from build123d import *

# Parameters (mm, degrees)
EXTRUDE1_DEPTH = 78
FILLET1_R      = 20
FILLET2_R      = 10
SKETCH3_R      = 7.5
EXTRUDE3_DEPTH = 6
FILLET3_R      = 30
SKETCH4_W      = 276.639181173
SKETCH4_H      = 310.570393871
EXTRUDE4_DEPTH = 79
SKETCH5_W      = 173
SKETCH5_H      = 59
EXTRUDE5_DEPTH = 65
EXTRUDE6_DEPTH = 94
SKETCH2_R      = 5
EXTRUDE2_DEPTH = 405
FILLET4_R      = 30
FILLET5_R      = 30


with BuildPart() as part:
    # Sketch1 → Extrude1 (new body)
    with BuildSketch(Plane(origin=(0, 0, 0), x_dir=(0, 0, -1), z_dir=(1, 0, 0))):
        Polygon((-38.878108718, 93.787762145), (-38.878108718, 8.787762145), (16.121891282, -76.212237855), (361.121891282, -76.212237855), (361.121891282, 123.787762145), (356.121891282, 123.787762145), (356.121891282, -71.212237855), (17.886597165, -71.212237855), (-33.878108718, 8.787762145), (-33.878108718, 93.787762145), align=None)
    extrude(amount=EXTRUDE1_DEPTH)

    # Fillet1
    fillet1_edges = [part.edges().sort_by_distance(p)[0] for p in [
        (39, -71.212237855, -356.121891282),
        (39, -76.212237855, -361.121891282),
    ]]
    fillet(fillet1_edges, radius=FILLET1_R)

    # Fillet2
    fillet2_edges = [part.edges().sort_by_distance(p)[0] for p in [
        (39, 8.787762145, 33.878108718),
        (39, -71.212237855, -17.886597165),
        (39, -76.212237855, -16.121891282),
        (39, 8.787762145, 38.878108718),
    ]]
    fillet(fillet2_edges, radius=FILLET2_R)

    # Sketch3 → Extrude3 (cut, through all)
    with BuildSketch(Plane(origin=(0, -71.212237855, 0), x_dir=(1, 0, 0), z_dir=(0, 1, 0))):
        with Locations((37.276272586, 74.00186583)):
            Circle(SKETCH3_R)
    extrude(amount=-EXTRUDE3_DEPTH, mode=Mode.SUBTRACT)

    # Fillet3
    fillet3_edges = [part.edges().sort_by_distance(p)[0] for p in [
        (0, 93.787762145, 36.378108718),
        (78, 93.787762145, 36.378108718),
    ]]
    fillet(fillet3_edges, radius=FILLET3_R)

    # Sketch4 → Extrude4 (cut, through all)
    with BuildSketch(Plane(origin=(78, 0, 0), x_dir=(0, 0, -1), z_dir=(1, 0, 0))):
        with Locations((344.441481869, 21.193022351)):
            Rectangle(SKETCH4_W, SKETCH4_H)
    extrude(amount=-EXTRUDE4_DEPTH, mode=Mode.SUBTRACT)

    # Sketch5 → Extrude5 (add)
    with BuildSketch(Plane(origin=(0, 0, -206.121891282), x_dir=(-1, 0, 0), z_dir=(0, 0, -1))):
        with Locations((-39, -46.712237855)):
            Rectangle(SKETCH5_W, SKETCH5_H)
    extrude(amount=EXTRUDE5_DEPTH)

    # Sketch6 → Extrude6 (add)
    with BuildSketch(Plane(origin=(0, 0, -271.121891282), x_dir=(-1, 0, 0), z_dir=(0, 0, -1))):
        with BuildLine():
            Line((-125.5, -76.212237855), (47.5, -76.212237855))
            Line((47.5, -76.212237855), (47.5, 101.787762145))
            ThreePointArc((47.5, 101.787762145), (32.855339059, 137.143101205), (-2.5, 151.787762145))
            Line((-2.5, 151.787762145), (-75.5, 151.787762145))
            ThreePointArc((-75.5, 151.787762145), (-110.855339059, 137.143101205), (-125.5, 101.787762145))
            Line((-125.5, 101.787762145), (-125.5, -76.212237855))
        make_face()
    extrude(amount=EXTRUDE6_DEPTH)

    # Sketch2 → Extrude2 (cut, through all)
    with BuildSketch(Plane.XY.offset(38.878108718)):
        with Locations((39, 78.787762145)):
            Circle(SKETCH2_R)
    extrude(amount=-EXTRUDE2_DEPTH, mode=Mode.SUBTRACT)

    # Fillet4
    fillet4_edges = [part.edges().sort_by_distance(p)[0] for p in [
        (125.5, -17.212237855, -238.621891282),
        (39, -17.212237855, -206.121891282),
        (-47.5, -17.212237855, -238.621891282),
        (39, -17.212237855, -271.121891282),
        (125.5, 42.287762145, -271.121891282),
        (-47.5, 42.287762145, -271.121891282),
        (-32.855339059, 137.143101205, -271.121891282),
        (39, 151.787762145, -271.121891282),
        (110.855339059, 137.143101205, -271.121891282),
    ]]
    fillet(fillet4_edges, radius=FILLET4_R)

    # Fillet5
    fillet5_edges = [part.edges().sort_by_distance(p)[0] for p in [
        (125.5, 12.787762145, -365.121891282),
        (39, -76.212237855, -365.121891282),
        (-47.5, 12.787762145, -365.121891282),
        (-32.855339059, 137.143101205, -365.121891282),
        (39, 151.787762145, -365.121891282),
        (110.855339059, 137.143101205, -365.121891282),
    ]]
    fillet(fillet5_edges, radius=FILLET5_R)


solid = part.part
Can you work these out from the model? Positions are in its coordinate system, mm. A direction names the side the tool comes from. Give positions to 0.01 mm unless a question says otherwise; leave off trailing zeros. Order: outer loops, then holes, each group sorted by start corner. A loop starts at its lowest first (then second) coordinate and runs counter-clockwise, first axis right, second up. Notation, with made-up numbers: (-8.75, 0.25) - (50.25, 0.25) arc R15 cw to (50.25, 26.25) - close; hole circle Ø5 at (24, -30). An arc over 180 degrees is marked (long way). Write each question's results on one line, items separated by ' | '.
1) On a 3-axis mill with a long thin cutter (end or side, diameter ignored), from which of +Z, -Z, +X, -X, +Y, -Y can I reach the whole of each face in a straight line? I mean faces 1 (the face through (38, -71.212, -116)), 2 (the face through (-38.945, 57.911, -280.143)), 3 (the face through (116.945, 56.665, -280.143)), 4 (the face through (38, 151.788, -318)), 5 (the face through (0, -73, -47)). Say none if no direction works.
Final values:
face 1: +X, -X, +Y | face 2: +Z, -X, +Y | face 3: +Z, +X, +Y | face 4: +Z, -Z, +X, -X, +Y | face 5: +Z, -X, +Y, -Y
2) If we mould it in two halves opening along Z, with no side actions, what happens to faces 6 (the face through (38.21, -8.66, -262.1)), 7 (the face through (39.546, -69.963, -18.487)), 8 (the face through (78, -73, -47)), 9 (the face through (37.79, -67.19, -356.57))? For each: pulls with the +Z half, pulls with the -Z half, needs draft (parallel to the pull), parting line crosses it, or undercut.
Final values:
face 6: undercut | face 7: undercut | face 8: needs draft | face 9: pulls with the -Z half
3) Suppose I cut it at A-A, the plane y = 35. Write out the boundary of the cut face in (x, z).
Final values:
outline: (-47.5, -335.12) arc R30 ccw to (-17.5, -365.12) - (95.5, -365.12) arc R30 ccw to (125.5, -335.12) - (125.5, -301.12) arc R30 ccw to (95.5, -271.12) - (-17.5, -271.12) arc R30 ccw to (-47.5, -301.12) - close; (0, 33.88) - (78, 33.88) - (78, 38.88) - (0, 38.88) - close
4) Suppose I cut it at D-D, the plane z = -146.5. Write out the boundary of the cut face in (x, y), then the cut area to 3 significant figures.
Final values:
outline: (0, -76.21) - (78, -76.21) - (78, -71.21) - (0, -71.21) - close | area: 390 mm^2
5) Suppose I cut it at B-B, the plane x = 39. Give the number of separate pieces and of enclosed holes in the cut face, then the cut area to 3 significant figures.
Final values:
separate pieces: 4 | enclosed holes: 0 | area: 25,400 mm^2
6) I'm going to push flat-ended pins straight in: pin 1 Ø1.5 at (x, z) = (22, -238) entering from +Y; pin 2 Ø4 at (x, z) = (36, 36) entering from +Y; pin 3 Ø1 at (x, y) = (92, 71) entering from +Z. Where does each tip first touch, or does it pass through?
Final values:
pin 1: stops at y = -17.21 | pin 2: stops at y = 93.79 | pin 3: stops at z = -271.12
7) Please list where these lines run through material, in increasing order: line 1 along Z through (x, y) = (10.5, 40.5); line 2 along Z through (x, y) = (-13.5, 91); line 3 along Y through (x, z) = (39, 37). Write a range as [from, to].
Final values:
line 1: z = [-365.12, -271.12], [33.88, 38.88] | line 2: z = [-365.12, -271.12] | line 3: y = [5.89, 73.79], [83.79, 93.79]
8) Suppose I cut it at C-C, the plane x = 64. Write out the boundary of the cut face in (y, z), then the cut area to 3 significant figures.
Final values:
outline: (-76.21, -335.12) arc R30 ccw to (-46.21, -365.12) - (121.79, -365.12) arc R30 ccw to (151.79, -335.12) - (151.79, -301.12) arc R30 ccw to (121.79, -271.12) - (12.79, -271.12) arc R30 cw to (-17.21, -241.12) - (-17.21, -236.12) arc R30 ccw to (-47.21, -206.12) - (-71.21, -206.12) - (-71.21, -23.33) arc R10 cw to (-66.64, -14.93) - (6.31, 32.27) arc R10 cw to (11.74, 33.88) - (89.16, 33.88) - (89.16, 38.88) - (11.74, 38.88) arc R10 ccw to (6.31, 37.27) - (-71.64, -13.17) arc R10 ccw to (-76.21, -21.56) - close | area: 26,400 mm^2
